Here's how the part is built. I have some questions about the finished solid (model axes, mm). A direction names the side the tool comes from. Coordinates: 2 decimals unless noted, no trailing zeros. Loops run counter-clockwise (first coordinate to the right, second up) from the corner with the lowest first, then second, coordinate; pieces in that order, holes last. Notation, with made-up numbers: (32.25, 17.5) - (36.25, 17.5) arc R20 cw to (36.25, 55.5) - close; hole circle Ø6 at (-1, -2). An arc over 180 degrees is marked (long way). Use a Markdown table: item, result.
```python
from build123d import *

# Parameters (mm, degrees)
SKETCH1_R           = 3
BOSS_EXTRUDE1_DEPTH = 3
SKETCH1_3_R         = 3
SKETCH1_3_R_2       = 1.600003175
BOSS_EXTRUDE2_DEPTH = 6
FILLET1_R           = 1
SKETCH2_R           = 2.55
BOSS_EXTRUDE3_DEPTH = 3
FILLET2_R           = 3


with BuildPart() as part:
    # Sketch1 → Boss-Extrude1 (new body)
    with BuildSketch(Plane.XY):
        with BuildLine():
            ThreePointArc((99.987500635, 4.00000762), (98.819645279, 1.180555381), (96.00019304, 0.012700025))
            Line((96.00019304, 0.012700025), (4.00000762, 0.012700025))
            ThreePointArc((4.00000762, 0.012700025), (1.180555381, 1.180555381), (0.012700025, 4.00000762))
            Line((0.012700025, 4.00000762), (0.012700025, 46.00009144))
            ThreePointArc((0.012700025, 46.00009144), (1.180555381, 48.819543679), (4.00000762, 49.987399035))
            Line((4.00000762, 49.987399035), (96.00019304, 49.987399035))
            ThreePointArc((96.00019304, 49.987399035), (98.819645279, 48.819543679), (99.987500635, 46.00009144))
            Line((99.987500635, 46.00009144), (99.987500635, 4.00000762))
        make_face()
        with Locations((95.0001905, 5.00001016)):
            Circle(SKETCH1_R, mode=Mode.SUBTRACT)
        with Locations((5.00001016, 5.00001016)):
            Circle(SKETCH1_R, mode=Mode.SUBTRACT)
        with Locations((95.0001905, 45.0000889)):
            Circle(SKETCH1_R, mode=Mode.SUBTRACT)
        with Locations((5.00001016, 45.0000889)):
            Circle(SKETCH1_R, mode=Mode.SUBTRACT)
    extrude(amount=BOSS_EXTRUDE1_DEPTH)

    # Sketch1<3> → Boss-Extrude2 (add)
    # profile 1 of 4: a face of its own
    with BuildSketch(Plane.XY):
        with Locations((5.00001016, 45.0000889)):
            Circle(SKETCH1_3_R)
        with Locations((5.00001016, 45.0000889)):
            Circle(SKETCH1_3_R_2, mode=Mode.SUBTRACT)
    # profile 2 of 4: a face of its own
    with BuildSketch(Plane.XY):
        with Locations((95.0001905, 45.0000889)):
            Circle(SKETCH1_3_R)
        with Locations((95.0001905, 45.0000889)):
            Circle(SKETCH1_3_R_2, mode=Mode.SUBTRACT)
    # profile 3 of 4: a face of its own
    with BuildSketch(Plane.XY):
        with Locations((95.0001905, 5.00001016)):
            Circle(SKETCH1_3_R)
        with Locations((95.0001905, 5.00001016)):
            Circle(SKETCH1_3_R_2, mode=Mode.SUBTRACT)
    # profile 4 of 4: a face of its own
    with BuildSketch(Plane.XY):
        with Locations((5.00001016, 5.00001016)):
            Circle(SKETCH1_3_R)
        with Locations((5.00001016, 5.00001016)):
            Circle(SKETCH1_3_R_2, mode=Mode.SUBTRACT)
    extrude(amount=BOSS_EXTRUDE2_DEPTH)

    # Fillet1
    fillet1_edges = [part.edges().sort_by_distance(p)[0] for p in [
        (92.0001905, 5.00001016, 3),
        (2.00001016, 5.00001016, 3),
        (92.0001905, 45.0000889, 3),
        (2.00001016, 45.0000889, 3),
    ]]
    fillet(fillet1_edges, radius=FILLET1_R)

    # Sketch2 → Boss-Extrude3 (add)
    # profile 1 of 4: a face of its own
    with BuildSketch(Plane.XY.offset(3)):
        with BuildLine():
            ThreePointArc((-4.987299975, 30.00004953), (-9.987299975, 25.00004953), (-4.987299975, 20.00004953))
            Line((-4.987299975, 20.00004953), (0.012700025, 20.00004953))
            Line((0.012700025, 20.00004953), (0.012700025, 25.00004953))
            Line((0.012700025, 25.00004953), (0.012700025, 30.00004953))
            Line((0.012700025, 30.00004953), (-4.987299975, 30.00004953))
        make_face()
        with Locations((-4.987299975, 25.00004953)):
            Circle(SKETCH2_R, mode=Mode.SUBTRACT)
    # profile 2 of 4: a face of its own
    with BuildSketch(Plane.XY.offset(3)):
        with BuildLine():
            Line((99.987500635, 30.00004953), (99.987500635, 25.00004953))
            Line((99.987500635, 25.00004953), (99.987500635, 20.00004953))
            Line((99.987500635, 20.00004953), (104.987500635, 20.00004953))
            ThreePointArc((104.987500635, 20.00004953), (109.987500635, 25.00004953), (104.987500635, 30.00004953))
            Line((104.987500635, 30.00004953), (99.987500635, 30.00004953))
        make_face()
        with Locations((104.987500635, 25.00004953)):
            Circle(SKETCH2_R, mode=Mode.SUBTRACT)
    # profile 3 of 4: a face of its own
    with BuildSketch(Plane.XY.offset(3)):
        with BuildLine():
            Line((45.00010033, 49.987399035), (50.00010033, 49.987399035))
            Line((50.00010033, 49.987399035), (55.00010033, 49.987399035))
            Line((55.00010033, 49.987399035), (55.00010033, 54.987399035))
            ThreePointArc((55.00010033, 54.987399035), (50.00010033, 59.987399035), (45.00010033, 54.987399035))
            Line((45.00010033, 54.987399035), (45.00010033, 49.987399035))
        make_face()
        with Locations((50.00010033, 54.987399035)):
            Circle(SKETCH2_R, mode=Mode.SUBTRACT)
    # profile 4 of 4: a face of its own
    with BuildSketch(Plane.XY.offset(3)):
        with BuildLine():
            Line((55.00010033, 0.012700025), (50.00010033, 0.012700025))
            Line((50.00010033, 0.012700025), (45.00010033, 0.012700025))
            Line((45.00010033, 0.012700025), (45.00010033, -4.987299975))
            ThreePointArc((45.00010033, -4.987299975), (50.00010033, -9.987299975), (55.00010033, -4.987299975))
            Line((55.00010033, -4.987299975), (55.00010033, 0.012700025))
        make_face()
        with Locations((50.00010033, -4.987299975)):
            Circle(SKETCH2_R, mode=Mode.SUBTRACT)
    extrude(amount=-BOSS_EXTRUDE3_DEPTH)

    # Fillet2
    fillet2_edges = [part.edges().sort_by_distance(p)[0] for p in [
        (99.987500635, 30.00004953, 1.5),
        (99.987500635, 20.00004953, 1.5),
        (55.00010033, 0.012700025, 1.5),
        (45.00010033, 0.012700025, 1.5),
        (0.012700025, 20.00004953, 1.5),
        (0.012700025, 30.00004953, 1.5),
        (55.00010033, 49.987399035, 1.5),
        (45.00010033, 49.987399035, 1.5),
    ]]
    fillet(fillet2_edges, radius=FILLET2_R)


solid = part.part
```
Q1. If we mould it in two halves opening along X, with no side actions, what happens to faces 1 (the face through (44.098, -0.843, 1.479)), 2 (the face through (4.792, 46.586, 2.958)), 3 (the face through (109.986, 24.89, 1.521)), 4 (the face through (93.4, 5.07, 2.96))? For each: pulls with the +X half, pulls with the -X half, needs draft (parallel to the pull), parting line crosses it, or undercut.
Check values:
| item | result |
|---|---|
| face 1 | pulls with the -X half |
| face 2 | undercut |
| face 3 | pulls with the +X half |
| face 4 | undercut |
Q2. Will these pins go through, and if not, where does the flat tip stop? P1, Ø1, axis at x = -4, z = 2, coming from the -Y side; P2, Ø6, axis at x = 104.99, y = 25, coming from the +Z side; P3, Ø1.5, axis at y = 13.5, z = 2, coming from the -X side.
Check values:
| item | result |
|---|---|
| P1 | y = 20 |
| P2 | z = 3 |
| P3 | x = 0.01 |
Q3. I want a section at C-C, the plane z = 1.15. Give the number of separate pieces and of enclosed holes in the cut face, then the cut area to 3 significant figures.
Check values:
| item | result |
|---|---|
| separate pieces | 1 |
| enclosed holes | 8 |
| area | 5,240 mm^2 |
Q4. Please list where these lines run through material, in increasing order: L1, parallel to X at y = -5, z = 1.05; L2, parallel to X at y = 53.5, z = 0.3; L3, parallel to Z at x = 46.5, y = 36. Write a range as from..to.
Check values:
| item | result |
|---|---|
| L1 | 45..47.45, 52.55..55 |
| L2 | 45..47.93, 52.07..55 |
| L3 | 0..3 |
Q5. I want a section at B-B, the plane y = 37. Write out the boundary of the cut face in (x, z).
Check values:
| item | result |
|---|---|
| outline | (0.01, 0) - (99.99, 0) - (99.99, 3) - (0.01, 3) - close |
Q6. Which directions (+Z, -Z, +X, -X, +Y, -Y) give clear straight access to the entire face, cutting with the end or side of a thin tool? Please do faces 5 (the face through (99.988, 11, 1)), 6 (the face through (6.3, 3.7, 6)), 7 (the face through (23, 49.987, 1)).
Check values:
| item | result |
|---|---|
| face 5 | +Z, -Z, +X, -Y |
| face 6 | +Z, +X, -X, +Y, -Y |
| face 7 | +Z, -Z, -X, +Y |
Q7. I want a section at A-A, the plane x = 22.5. Write out the boundary of the cut face in (y, z), then the cut area to 3 significant figures.
Check values:
| item | result |
|---|---|
| outline | (0.01, 0) - (49.99, 0) - (49.99, 3) - (0.01, 3) - close |
| area | 150 mm^2 |
